```python
from build123d import *

# Parameters (mm, degrees)
SKETCH1_R           = 2.15
BOSS_EXTRUDE1_DEPTH = 4


with BuildPart() as part:
    # Sketch1 → Boss-Extrude1 (new body)
    with BuildSketch(Plane.XY):
        with BuildLine():
            Line((-3.1, -7), (-3.1, 0))
            ThreePointArc((-3.1, 0), (0, 3.1), (3.1, 0))
            Line((3.1, 0), (3.1, -7))
            Line((3.1, -7), (35.005, -7))
            Line((35.005, -7), (35.005, 0))
            ThreePointArc((35.005, 0), (38.105, 3.1), (41.205, 0))
            Line((41.205, 0), (41.205, -7))
            Line((41.205, -7), (45.064925835, -7))
            Line((45.064925835, -7), (45.064925835, -0.747952118))
            ThreePointArc((45.064925835, -0.747952118), (43.312478508, 4.677837918), (38.105, 7))
            Line((38.105, 7), (-12.106664199, 7))
            ThreePointArc((-12.106664199, 7), (-15.606664199, 6.062177826), (-18.168842026, 3.5))
            Line((-18.168842026, 3.5), (-44.843842026, -42.702455292))
            Line((-44.843842026, -42.702455292), (-38.781664199, -46.202455292))
            ThreePointArc((-38.781664199, -46.202455292), (-38.263860854, -48.590239831), (-40.690427119, -48.875566784))
            Line((-40.690427119, -48.875566784), (-46.478523985, -45.5338075))
            Line((-46.478523985, -45.5338075), (-60.668842026, -70.112159322))
            ThreePointArc((-60.668842026, -70.112159322), (-60.968543293, -72.388616457), (-59.570765814, -74.210235533))
            Line((-59.570765814, -74.210235533), (-48.918653348, -80.360235533))
            ThreePointArc((-48.918653348, -80.360235533), (-46.642196213, -80.659936801), (-44.820577137, -79.262159322))
            Line((-44.820577137, -79.262159322), (-3.1, -7))
        make_face()
        with Locations((-52.106664199, -69.282032303)):
            Circle(SKETCH1_R, mode=Mode.SUBTRACT)
        with Locations((-27.106664199, -25.980762114)):
            Circle(SKETCH1_R, mode=Mode.SUBTRACT)
    extrude(amount=BOSS_EXTRUDE1_DEPTH)


solid = part.part
```
Part model, mm, in its own coordinate system. A direction names the side the tool comes from. Round coordinates to 2 decimals unless told otherwise and drop trailing zeros. Write each loop counter-clockwise with the first axis right and the second up, starting at its lowest first coordinate (ties: lowest second). Pieces come first, ordered by that corner, then holes. Notation, with made-up numbers: M 5,17.5 L 48,17.5 A11 cw 48,38.5 Z; hole C 27.5,13 d5. An arc over 180 degrees is marked long. Answer as CSV lines item,"result". Start each with the question number.
1) Band-saw the part on A-A (z = 0.85). List the corners of the cut face in (x, y) (3 decimals), then the cut area to 3 significant figures.
2) Drop flat-ended pins along their axis: pin 1 (2 mm diameter, centred on y = -65.5, z = 3, fed in from +X); pin 2 (1.2 mm diameter, centred on y = -4.5, z = 1.5, fed in from +X); pin 3 (1.2 mm diameter, centred on y = -5, z = 2, fed in from -X); pin 4 (2.5 mm diameter, centred on x = -27.11, y = -25.98, fed in from +Z). Give the stop position or say it passes through.
3) Band-saw the part on C-C (y = -35.5). List the corners of the cut face in (x, z).
4) Band-saw the part on B-B (x = 0). List the corners of the cut face in (y, z), then the cut area to 3 significant figures.
5) Mould opens along X. For faces 1 (the face through (-60.977, -72.357, 1.972)), 2 (the face through (-0.1, 3.1, 2)), 3 (the face through (43, -7, 2)), 4 (the face through (45.065, -4, 2)) say: +X half, -X half, draft (parallel to the pull), parting line (faces both ways), or undercut.
6) Which spindle directions (+Z, -Z, +X, -X, +Y, -Y) get a long thin tool onto all of the face, cutting with end or side? Do faces 5 (the face through (-41.9, -44.4, 2)), 6 (the face through (19, -7, 2)), 7 (the face through (41.205, -3, 2)). Say none if no direction does.
7) Drill centre lines: L1, parallel to X at y = -1.5, z = 1.1 (3 decimals); L2, parallel to X at y = -3, z = 1.05 (3 decimals); L3, parallel to Y at x = 5, z = 0.95. Where is each one in solid material? Low to high.
Worked out:
1,outline,"M -60.669,-70.112 A3 ccw -59.571,-74.21 L -48.919,-80.36 A3 ccw -44.821,-79.262 L -3.1,-7 L -3.1,0 A3.1 cw 3.1,0 L 3.1,-7 L 35.005,-7 L 35.005,0 A3.1 cw 41.205,0 L 41.205,-7 L 45.065,-7 L 45.065,-0.748 A7 ccw 38.105,7 L -12.107,7 A7 ccw -18.169,3.5 L -44.844,-42.702 L -38.782,-46.202 A1.65 cw long -40.69,-48.876 L -46.479,-45.534 Z; hole C -52.107,-69.282 d4.3; hole C -27.107,-25.981 d4.3"
1,area,"2,210 mm²"
2,pin 1,"x = -36.3"
2,pin 2,"x = 45.06"
2,pin 3,"x = -23.42"
2,pin 4,"through"
3,outline,"M -40.69,0 L -19.55,0 L -19.55,4 L -40.69,4 Z"
4,outline,"M 3.1,0 L 7,0 L 7,4 L 3.1,4 Z"
4,area,"15.6 mm²"
5,face 1,"-X half"
5,face 2,"undercut"
5,face 3,"draft"
5,face 4,"+X half"
6,face 5,"+Z, -Z"
6,face 6,"+Z, -Z, +X, -Y"
6,face 7,"+Z, -Z, -Y"
7,L1,"-21.056 to -3.1, 3.1 to 35.005, 41.205 to 45.065"
7,L2,"-21.922 to -3.1, 3.1 to 35.005, 41.205 to 45.065"
7,L3,"-7 to 7"
